```python
from build123d import *

# Parameters (mm, degrees)
SKETCH1_W                    = 1000
SKETCH1_H                    = 200
BASE_FLANGE1_DEPTH           = 3
EDGE_FLANGE1_STRIP_W         = 52
EDGE_FLANGE1_STRIP_H         = 3
EDGE_FLANGE1_STRIP_CUT_DEPTH = 200
EDGE_FLANGE1_DEPTH           = 200
EDGE_FLANGE1_FLAT_DEPTH      = 3
EDGE_FLANGE2_STRIP_W         = 52
EDGE_FLANGE2_STRIP_H         = 3
EDGE_FLANGE2_STRIP_CUT_DEPTH = 200
EDGE_FLANGE2_DEPTH           = 200
EDGE_FLANGE2_FLAT_DEPTH      = 3
SKETCH13_R                   = 10
CUT_EXTRUDE1_DEPTH           = 1010.189774027


# Sheet-metal steps are written as plain solids
with BuildPart() as part:
    # Sketch1 → Base-Flange1 (new body)
    with BuildSketch(Plane(origin=(0, 0, 0), x_dir=(1, 0, 0), z_dir=(0, 1, 0))):
        Rectangle(SKETCH1_W, SKETCH1_H)
    extrude(amount=-BASE_FLANGE1_DEPTH)

    # Edge-Flange1 strip (across the edge) → Edge-Flange1 strip cut (cut)
    with BuildSketch(Plane(origin=(-500, 0, -100), x_dir=(1, 0, 0), z_dir=(0, 0, 1))):
        with Locations((-3, -1.5)):
            Rectangle(EDGE_FLANGE1_STRIP_W, EDGE_FLANGE1_STRIP_H)
    extrude(amount=EDGE_FLANGE1_STRIP_CUT_DEPTH, mode=Mode.SUBTRACT)

    # Edge-Flange1 bend section (across the edge) → Edge-Flange1 (add)
    with BuildSketch(Plane(origin=(-500, 0, -100), x_dir=(1, 0, 0), z_dir=(0, 0, 1))):
        with BuildLine():
            Line((0, 20), (3, 20))
            ThreePointArc((3, 20), (8.857864376, 5.857864376), (23, 0))
            Line((23, 0), (23, -3))
            ThreePointArc((23, -3), (6.736544033, 3.736544033), (0, 20))
        make_face()
    extrude(amount=EDGE_FLANGE1_DEPTH)

    # Edge-Flange1 profile (on flange) → Edge-Flange1 flat (add)
    with BuildSketch(Plane.ZY.offset(500)):
        with BuildLine():
            Line((-100, 92), (-100, 20))
            Line((-100, 20), (100, 20))
            Line((100, 20), (100, 57))
            ThreePointArc((100, 57), (89.748737342, 81.748737342), (65, 92))
            Line((65, 92), (-100, 92))
        make_face()
    extrude(amount=-EDGE_FLANGE1_FLAT_DEPTH)

    # Edge-Flange2 strip (across the edge) → Edge-Flange2 strip cut (cut)
    with BuildSketch(Plane(origin=(500, 0, 100), x_dir=(-1, 0, 0), z_dir=(0, 0, -1))):
        with Locations((-3, -1.5)):
            Rectangle(EDGE_FLANGE2_STRIP_W, EDGE_FLANGE2_STRIP_H)
    extrude(amount=EDGE_FLANGE2_STRIP_CUT_DEPTH, mode=Mode.SUBTRACT)

    # Edge-Flange2 bend section (across the edge) → Edge-Flange2 (add)
    with BuildSketch(Plane(origin=(500, 0, 100), x_dir=(-1, 0, 0), z_dir=(0, 0, -1))):
        with BuildLine():
            Line((0, 20), (3, 20))
            ThreePointArc((3, 20), (8.857864376, 5.857864376), (23, 0))
            Line((23, 0), (23, -3))
            ThreePointArc((23, -3), (6.736544033, 3.736544033), (0, 20))
        make_face()
    extrude(amount=EDGE_FLANGE2_DEPTH)

    # Edge-Flange2 profile (on flange) → Edge-Flange2 flat (add)
    with BuildSketch(Plane(origin=(500, 0, 0), x_dir=(0, 0, -1), z_dir=(1, 0, 0))):
        with BuildLine():
            Line((100, 92), (-65, 92))
            ThreePointArc((-65, 92), (-89.748737342, 81.748737342), (-100, 57))
            Line((-100, 57), (-100, 20))
            Line((-100, 20), (100, 20))
            Line((100, 20), (100, 92))
        make_face()
    extrude(amount=-EDGE_FLANGE2_FLAT_DEPTH)

    # Sketch13 → Cut-Extrude1 (cut, through all)
    with BuildSketch(Plane.ZY.offset(500)):
        with Locations(Location((60, 57, 0), (0, 0, 270))):
            Circle(SKETCH13_R)
        Polygon((-100, 20), (-50, 92.245135124), (-100, 92), align=None)
    extrude(amount=-CUT_EXTRUDE1_DEPTH, mode=Mode.SUBTRACT)


solid = part.part
```
Can you work these out from the model? Positions are in its coordinate system, mm. A direction names the side the tool comes from. Coordinates: 2 decimals unless noted, no trailing zeros. Order: outer loops, then holes, each group sorted by start corner. A loop starts at its lowest first (then second) coordinate and runs counter-clockwise, first axis right, second up.
1. If we section it at D-D (z = -80): Please give me the cut outline in (x, y).
2. For faces 5 (the face through (-498.52, 55.5, -75.43)), 6 (the face through (497, 57, 1)), which set-ups out of +Z, -Z, +X, -X, +Y, -Y let a thin tool reach every point of the face, with its end or its side?
3. If we section it at C-C (x = 99): Please give me the cut outline in (y, z).
4. I need wall thicknesses on line 1 (X direction, y = 50.5, z = 21.5); line 2 (Z direction, x = -498.7, y = 57); line 3 (Y direction, x = -415, z = -87). Which ranges of each line are inside material? Lowest first, please.
5. I'm going to push flat-ended pins straight in: pin 1 (3 mm diameter, centred on y = 13, z = -73.5, fed in from -X); pin 2 (1 mm diameter, centred on x = -363.5, z = -42.5, fed in from +Y). Where does each tip first touch, or does it pass through?
6. If we section it at A-A (y = 11): Please give me the cut outline in (x, z).
7. If we section it at B-B (z = -8): Please give me the cut outline in (x, y).
8. Thinking about a two-plate mould opening in Z: for faces 1 (the face through (493.084, 3.559, 1.4)), 2 (the face through (-499, 65, 54)), 3 (the face through (498.48, 55.5, -75.43)), 4 (the face through (498, 65, 54)), which applies, +Z half, -Z half, draft (parallel to the pull), parting line (faces both ways), or undercut?
Entries:
1. outline: (-500, 20) arc R23 ccw to (-477, -3) - (477, -3) arc R23 ccw to (500, 20) - (500, 48.9) - (497, 48.9) - (497, 20) arc R20 cw to (477, 0) - (-477, 0) arc R20 cw to (-497, 20) - (-497, 48.9) - (-500, 48.9) - close
2. face 5: -Z, +X, -X, +Y
2. face 6: +Z, -Z, +Y
3. outline: (-3, -100) - (0, -100) - (0, 100) - (-3, 100) - close
4. line 1: x = -500 to -497, 497 to 500
4. line 2: z = -74.39 to 50, 70 to 100
4. line 3: y = -3 to 0
5. pin 1: stops at x = -499.33
5. pin 2: stops at y = 0
6. outline: (-498.17, -100) - (-494.86, -100) - (-494.86, 100) - (-498.17, 100) - close; (494.86, -100) - (498.17, -100) - (498.17, 100) - (494.86, 100) - close
7. outline: (-500, 20) arc R23 ccw to (-477, -3) - (477, -3) arc R23 ccw to (500, 20) - (500, 92) - (497, 92) - (497, 20) arc R20 cw to (477, 0) - (-477, 0) arc R20 cw to (-497, 20) - (-497, 92) - (-500, 92) - close
8. face 1: draft
8. face 2: undercut
8. face 3: -Z half
8. face 4: undercut
